Source: CAD feature listing. Evaluate the final solid. Frame: model axes, mm. Face numbers are marked on the shaded views. A direction names the side the tool comes from. Round coordinates to 2 decimals unless told otherwise and drop trailing zeros. Order: outer loops, then holes, each group sorted by start corner. A loop starts at its lowest first (then second) coordinate and runs counter-clockwise, first axis right, second up. Notation, with made-up numbers: (-4.75, 10.5) -> (14.25, 10.5) arc R13 cw to (14.25, 14.5) -> close; hole circle Ø11 at (58.5, -13). An arc over 180 degrees is marked (long way). Answer as CSV lines item,"result". Start each with the question number.
(1) Section query A-A (x = 0). Output: boundary loops of the cut face in (y, z) (3 decimals), plus the area to 3 significant figures.
(2) Set-up query: the marked faces 1, 2, 3 and 4. Return all of +Z, -Z, +X, -X, +Y, -Y with unobstructed straight access to the full face (end or side cutting, diameter ignored); none if empty.
(3) Section query C-C (y = -7). Output: boundary loops of the cut face in (x, z), plus the area to 3 significant figures.
(4) Contact query for a flat-ended pin moving along its axis: P1, Ø1, axis at y = -7, z = 3, coming from the -X side. Output: stop coordinate, or through.
(5) Line query: line 1 along Y through (x, z) = (0, 0.65) (3 decimals); line 2 along Y through (x, z) = (0, 4.35) (3 decimals); line 3 along Y through (x, z) = (-11.75, 3.7). Output: solid intervals per line, ascending. Write a range as from..to.
(6) Section query B-B (y = 7.75). Output: boundary loops of the cut face in (x, z).
(7) Pull-direction query (Y, two-part tool) for the marked faces 5, 6, 7 and 8; classes: +Y half, -Y half, draft (parallel to the pull), parting line (faces both ways), or undercut.
```python
from build123d import *

# Parameters (mm, degrees)
CROQUIS1_R              = 15
CROQUIS1_R_2            = 1.5
SALIENTE_EXTRUIR1_DEPTH = 5
CORTAR_EXTRUIR1_DEPTH   = 22.794494718
MATRIZC1_COUNT          = 13
CROQUIS3_R              = 5
CORTAR_EXTRUIR2_DEPTH   = 2.5


with BuildPart() as part:
    # Croquis1 → Saliente-Extruir1 (new body)
    with BuildSketch(Plane.XY):
        Circle(CROQUIS1_R)
        Circle(CROQUIS1_R_2, mode=Mode.SUBTRACT)
    extrude(amount=SALIENTE_EXTRUIR1_DEPTH)

    # Croquis2 → Cortar-Extruir1 (cut, through all)
    with BuildSketch(Plane.XY.offset(5)):
        with BuildLine():
            ThreePointArc((2.827423232, 14.731112581), (0, 15), (-2.827423232, 14.731112581))
            ThreePointArc((-2.827423232, 14.731112581), (-1.836024404, 13.60728926), (-1.478404899, 12.151968408))
            ThreePointArc((-1.478404899, 12.151968408), (-1.151515386, 11.338657004), (-0.612545475, 10.64739466))
            ThreePointArc((-0.612545475, 10.64739466), (0, 10.665), (0.612545475, 10.64739466))
            ThreePointArc((0.612545475, 10.64739466), (1.320743225, 11.678795886), (1.57, 12.904847926))
            ThreePointArc((1.57, 12.904847926), (2.032147713, 13.93266315), (2.827423232, 14.731112581))
        make_face()
    cortar_extruir1 = extrude(amount=-CORTAR_EXTRUIR1_DEPTH, mode=Mode.SUBTRACT)

    # MatrizC1: Cortar-Extruir1 ×13 about axis
    matrizc1_axis = Axis((0, 0, 0), (0, 0, 1))
    for i in range(1, MATRIZC1_COUNT):
        add(cortar_extruir1.rotate(matrizc1_axis, i * 360 / MATRIZC1_COUNT), mode=Mode.SUBTRACT)

    # Croquis3 → Cortar-Extruir2 (cut)
    with BuildSketch(Plane.XY.offset(5)):
        Circle(CROQUIS3_R)
    extrude(amount=-CORTAR_EXTRUIR2_DEPTH, mode=Mode.SUBTRACT)


solid = part.part
```
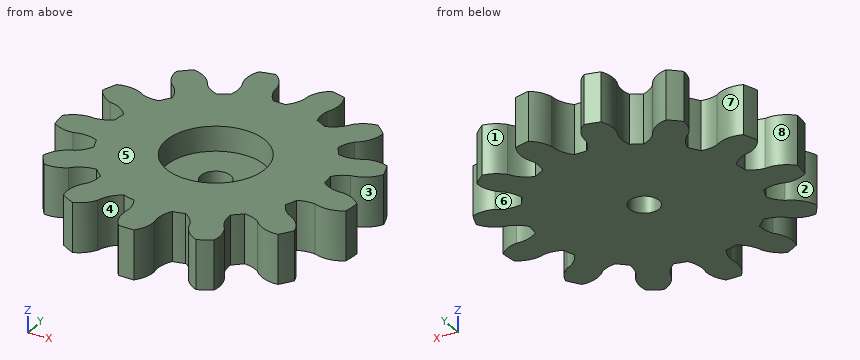
Answer block:
1,outline,"(-15, 0) -> (-1.5, 0) -> (-1.5, 2.5) -> (-5, 2.5) -> (-5, 5) -> (-15, 5) -> close; (1.5, 0) -> (10.665, 0) -> (10.665, 5) -> (5, 5) -> (5, 2.5) -> (1.5, 2.5) -> close"
1,area,"95.8 mm2"
2,face 1,"+Z, -Z, +Y"
2,face 2,"+Z, -Z, -X"
2,face 3,"+Z, -Z, +X"
2,face 4,"+Z, -Z, -Y"
3,outline,"(-12.41, 0) -> (12.41, 0) -> (12.41, 5) -> (-12.41, 5) -> close"
3,area,"124 mm2"
4,P1,"x = -12.66"
5,line 1,"-15..-1.5, 1.5..10.665"
5,line 2,"-15..-5, 5..10.665"
5,line 3,"-9.16..-6.23, -2.91..0.1, 2.88..6.12"
6,outline,"(-8.88, 0) -> (8.88, 0) -> (8.88, 5) -> (-8.88, 5) -> close"
7,face 5,"draft"
7,face 6,"undercut"
7,face 7,"+Y half"
7,face 8,"undercut"
